```python
from build123d import *

# Parameters (mm, degrees)
BOSS_EXTRUDE1_DEPTH = 8
SKETCH2_R           = 2.5
BOSS_EXTRUDE2_DEPTH = 3
SKETCH3_R           = 1.3
BOSS_EXTRUDE3_DEPTH = 3


with BuildPart() as part:
    # Sketch1 → Boss-Extrude1 (new body)
    with BuildSketch(Plane.XY):
        with BuildLine():
            Line((128.959100066, 33.628624999), (133.959100066, 33.628624999))
            Line((133.959100066, 33.628624999), (133.959100066, -45.656116492))
            Line((133.959100066, -45.656116492), (128.959100066, -45.656116492))
            add(Edge.make_bspline(
                [(113.496599029, -53.92747215), (114.973875685, -53.76034768), (116.389465073, -53.408303088), (118.438931288, -52.658652366), (119.109837198, -52.372048444), (120.430638868, -51.735858399), (121.082915856, -51.384782434), (122.988929436, -50.267489711), (124.197203446, -49.437169981), (126.541735842, -47.677906536), (127.677620036, -46.748450374), (128.850515141, -45.74891878), (128.904828159, -45.702543351), (128.959100066, -45.656116492)],
                knots=[0, 0, 0, 0, 0.125, 0.125, 0.1875, 0.1875, 0.25, 0.25, 0.375, 0.375, 0.5, 0.5, 0.506074438, 0.506074438, 0.506074438, 0.506074438], degree=3))
            Line((113.496599029, -53.92747215), (-75.963345356, -63.503442328))
            add(Edge.make_bspline(
                [(-96.040899934, -41.829259963), (-95.798899268, -42.093160096), (-95.56197213, -42.362136183), (-94.03954966, -44.156758027), (-92.923608678, -45.792412437), (-90.858487716, -49.170948695), (-89.911065512, -50.914960796), (-88.457766632, -53.51029646), (-87.967520262, -54.371999904), (-86.940892781, -56.06392928), (-86.404912323, -56.894254814), (-85.530671439, -58.091259413), (-85.227414802, -58.482089731), (-84.588818098, -59.241614046), (-84.254184704, -59.609132259), (-83.204929916, -60.651600397), (-82.440569541, -61.270576891), (-81.160629249, -62.042718444), (-80.719255742, -62.269433113), (-79.817314106, -62.660888928), (-79.3554021, -62.826549047), (-77.940467092, -63.243286827), (-76.954208328, -63.414201398), (-75.963345356, -63.503442328)],
                knots=[0.352672192, 0.352672192, 0.352672192, 0.352672192, 0.375, 0.375, 0.5, 0.5, 0.625, 0.625, 0.6875, 0.6875, 0.75, 0.75, 0.78125, 0.78125, 0.8125, 0.8125, 0.875, 0.875, 0.90625, 0.90625, 0.9375, 0.9375, 1, 1, 1, 1], degree=3))
            Line((-96.040899934, -41.829259963), (-101.040899934, -41.829259963))
            Line((-101.040899934, -41.829259963), (-101.040899934, 29.801740739))
            Line((-101.040899934, 29.801740739), (-96.040899934, 29.801740739))
            add(Edge.make_bspline(
                [(-75.963345356, 51.475952827), (-76.969760945, 51.385311169), (-77.956664013, 51.213742336), (-79.395866789, 50.78571401), (-79.86970863, 50.613871194), (-80.796837185, 50.204577199), (-81.240590365, 49.971323111), (-82.089787414, 49.449496549), (-82.495246976, 49.160946736), (-83.271465049, 48.533739024), (-83.643007435, 48.194375714), (-84.708444042, 47.116795042), (-85.333215001, 46.343374139), (-86.491296884, 44.737676097), (-87.023827607, 43.904896882), (-88.044872363, 42.211012893), (-88.533034054, 41.34968138), (-89.982900727, 38.756279626), (-90.93240726, 37.013628654), (-92.999467157, 33.650383947), (-94.114586107, 32.031232641), (-95.60337212, 30.287705281), (-95.819744565, 30.042891916), (-96.040899934, 29.801740739)],
                knots=[0, 0, 0, 0, 0.0625, 0.0625, 0.09375, 0.09375, 0.125, 0.125, 0.15625, 0.15625, 0.1875, 0.1875, 0.25, 0.25, 0.3125, 0.3125, 0.375, 0.375, 0.5, 0.5, 0.625, 0.625, 0.645748558, 0.645748558, 0.645748558, 0.645748558], degree=3))
            Line((-75.963345356, 51.475952827), (113.496599029, 41.899982649))
            add(Edge.make_bspline(
                [(128.959100066, 33.628624999), (128.913387154, 33.667730585), (127.751192536, 34.660386778), (126.568806099, 35.629041088), (124.805320754, 36.953884089), (124.207009004, 37.38378621), (122.992052543, 38.206145046), (122.374602128, 38.599251589), (120.484333172, 39.709851881), (119.174169326, 40.359663675), (117.093195419, 41.124643977), (116.387101294, 41.341482025), (114.957490187, 41.687263925), (114.232477088, 41.816732683), (113.496599029, 41.899982649)],
                knots=[0.494878569, 0.494878569, 0.494878569, 0.494878569, 0.5, 0.625, 0.625, 0.6875, 0.6875, 0.75, 0.75, 0.875, 0.875, 0.9375, 0.9375, 1, 1, 1, 1], degree=3))
        make_face()
    extrude(amount=BOSS_EXTRUDE1_DEPTH)

    # Sketch2 → Boss-Extrude2 (add)
    with BuildSketch(Plane.XY.offset(8)):
        with Locations((-86.273928885, 22.986240388)):
            Circle(SKETCH2_R)
        with Locations((-78.273928885, 36.986240388)):
            Circle(SKETCH2_R)
        with Locations((-20.273928885, 36.986240388)):
            Circle(SKETCH2_R)
        with Locations((-0.273928885, 22.986240388)):
            Circle(SKETCH2_R)
        with Locations((-0.273928885, -35.013759612)):
            Circle(SKETCH2_R)
        with Locations((-20.273928885, -49.013759612)):
            Circle(SKETCH2_R)
        with Locations((-78.273928885, -49.013759612)):
            Circle(SKETCH2_R)
        with Locations((-86.273928885, -35.013759612)):
            Circle(SKETCH2_R)
    extrude(amount=BOSS_EXTRUDE2_DEPTH)

    # Sketch3 → Boss-Extrude3 (add)
    with BuildSketch(Plane.XY.offset(11)):
        with Locations((-86.273928885, 22.986240388)):
            Circle(SKETCH3_R)
        with Locations((-78.273928885, 36.986240388)):
            Circle(SKETCH3_R)
        with Locations((-20.273928885, 36.986240388)):
            Circle(SKETCH3_R)
        with Locations((-0.273928885, 22.986240388)):
            Circle(SKETCH3_R)
        with Locations((-0.273928885, -35.013759612)):
            Circle(SKETCH3_R)
        with Locations((-20.273928885, -49.013759612)):
            Circle(SKETCH3_R)
        with Locations((-78.273928885, -49.013759612)):
            Circle(SKETCH3_R)
        with Locations((-86.273928885, -35.013759612)):
            Circle(SKETCH3_R)
    extrude(amount=BOSS_EXTRUDE3_DEPTH)


solid = part.part
```
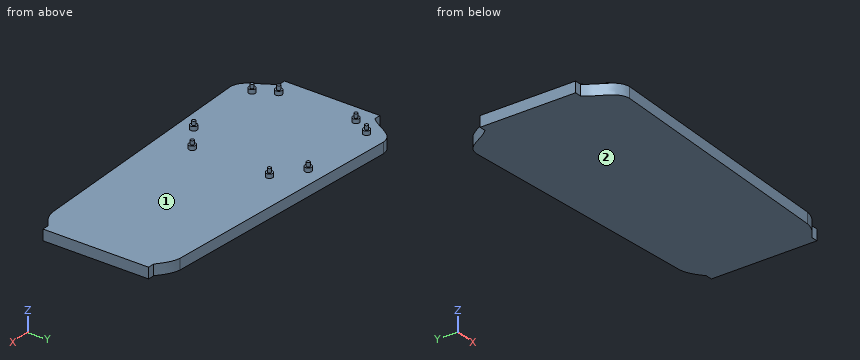
The model under review builds one solid part; all positions refer to its coordinate system, in mm. Face numbers are marked on the shaded views. Coordinates: 2 decimals unless noted, no trailing zeros. Write each loop counter-clockwise with the first axis right and the second up, starting at its lowest first coordinate (ties: lowest second). Pieces come first, ordered by that corner, then holes.
1) We need section B-B on x = 88.5. State the section outline as (y, z) points, then the cut area to 3 significant figures.
2) Clearance check with flat-ended pins moving along their axes: pin 1 Ø5.5 at (x, z) = (130.5, 4.5) entering from +Y; pin 2 Ø6 at (x, y) = (98, -29.5) entering from +Z; pin 3 Ø1 at (x, z) = (87.5, 2) entering from +Y. State where each tip first meets the part, or that it passes through.
3) To check wall thickness, follow probe 1 along Z at (x, y) = (-21, 13.5); probe 2 along Y at (x, z) = (-14.5, 1.75); probe 3 along X at (y, z) = (-42, 5.5). State the ranges of each line that lie inside material, in increasing order.
4) The part is to be moulded in two halves that separate along Z. For the marked faces 1 and 2, say which applies: pulls with the +Z half, pulls with the -Z half, needs draft (parallel to the pull), parting line crosses it, or undercut.
5) We need section A-A on y = -27. State the section outline as (x, z) points.
Answer list:
1. outline: (-55.19, 0) - (43.16, 0) - (43.16, 8) - (-55.19, 8) - close
1. area: 787 mm2
2. pin 1: stops at y = 34.65
2. pin 2: stops at z = 8
2. pin 3: stops at y = 43.24
3. probe 1: z = 0 to 8
3. probe 2: y = -60.4 to 48.37
3. probe 3: x = -95.89 to 133.96
4. face 1: pulls with the +Z half
4. face 2: pulls with the -Z half
5. outline: (-101.04, 0) - (133.96, 0) - (133.96, 8) - (-101.04, 8) - close
